Could you check a few things on this model? Use its own coordinates, in mm. Give positions to 0.01 mm unless a question says otherwise; leave off trailing zeros. Loops run counter-clockwise (first coordinate to the right, second up) from the corner with the lowest first, then second, coordinate; pieces in that order, holes last. Notation, with made-up numbers: (-15.5, -14.5) - (22.5, -14.5) arc R24 ccw to (22.5, -4.5) - close; hole circle Ø3 at (55.5, 45.5). An arc over 180 degrees is marked (long way). One line per item, written item: value. Start each with the question number.
Q1. I'm going to push flat-ended pins straight in: P1, Ø4, axis at y = -227.5, z = 155.5, coming from the -X side; P2, Ø2, axis at x = -122.5, z = 405.5, coming from the +Y side; P3, Ø6, axis at x = -8, y = 129.5, coming from the -Z side. Where does each tip first touch, or does it pass through?
Q2. If I drill on line 1 (Z direction, x = 214, y = 232.5); line 2 (X direction, y = -24.5, z = 295.5); line 3 (Y direction, x = -209, z = 122.5), over which ranges is the centre line in solid material (lowest first)? Write a range as from..to.
Q3. I want a section at B-B (x = 51.5). Please give me the cut outline in (y, z).
Q4. If we mould it in two halves opening along Y, with no side actions, what happens to faces 1 (the face through (-10.99, -249.76, 138.75)), 2 (the face through (-74, -239, 12))? For each: released by +Y, released by -Y, zero draft, split by the parting line, or undercut.
Q5. I want a section at C-C (z = 111). Please give me the cut outline in (x, y).
Q6. I want a section at A-A (y = 0). Please give me the cut outline in (x, z).
```python
from build123d import *

# Parameters (mm, degrees)
SKETCH1_R           = 325
SKETCH1_R_2         = 6
SKETCH1_R_3         = 244
BOSS_EXTRUDE1_DEPTH = 12


with BuildPart() as part:
    # Sketch1 → Boss-Extrude1 (new body)
    with BuildSketch(Plane.XY):
        Circle(SKETCH1_R)
        with Locations((0, 287.5)):
            Circle(SKETCH1_R_2, mode=Mode.SUBTRACT)
        with Locations((168.988260034, 232.592385883)):
            Circle(SKETCH1_R_2, mode=Mode.SUBTRACT)
        with Locations((273.428748435, 88.842385883)):
            Circle(SKETCH1_R_2, mode=Mode.SUBTRACT)
        with Locations((273.428748435, -88.842385883)):
            Circle(SKETCH1_R_2, mode=Mode.SUBTRACT)
        with Locations((168.988260034, -232.592385883)):
            Circle(SKETCH1_R_2, mode=Mode.SUBTRACT)
        with Locations((0, -287.5)):
            Circle(SKETCH1_R_2, mode=Mode.SUBTRACT)
        with Locations((-168.988260034, -232.592385883)):
            Circle(SKETCH1_R_2, mode=Mode.SUBTRACT)
        with Locations((-273.428748435, -88.842385883)):
            Circle(SKETCH1_R_2, mode=Mode.SUBTRACT)
        with Locations((-273.428748435, 88.842385883)):
            Circle(SKETCH1_R_2, mode=Mode.SUBTRACT)
        with Locations((-168.988260034, 232.592385883)):
            Circle(SKETCH1_R_2, mode=Mode.SUBTRACT)
        Circle(SKETCH1_R_3, mode=Mode.SUBTRACT)
    extrude(amount=BOSS_EXTRUDE1_DEPTH)

    # Sketch4 → Revolve2 (revolve)
    with BuildSketch(Plane(origin=(0, 0, 0), x_dir=(0, 0, -1), z_dir=(1, 0, 0))):
        with BuildLine():
            Line((-12, 250), (-262, 250))
            ThreePointArc((-262, 250), (-438.776695297, 176.776695297), (-512, 0))
            Line((-512, 0), (-506, 0))
            ThreePointArc((-506, 0), (-434.53405461, 172.53405461), (-262, 244))
            Line((-262, 244), (-12, 244))
            Line((-12, 244), (-12, 250))
        make_face()
    revolve(axis=Axis((0, 0, 12), (0, 0, 1)))


solid = part.part
```
Worked answers:
1. P1: stops at x = -107.93
1. P2: stops at y = 165.16
1. P3: stops at z = 466.73
2. line 1: z = 0..12
2. line 2: x = -246.53..-240.44, 240.44..246.53
2. line 3: y = -137.18..-125.92, 125.92..137.18
3. outline: (-320.89, 0) - (-238.5, 0) - (-238.5, 262) arc R238.5 cw to (238.5, 262) - (238.5, 0) - (320.89, 0) - (320.89, 12) - (244.64, 12) - (244.64, 262) arc R244.64 ccw to (-244.64, 262) - (-244.64, 12) - (-320.89, 12) - close
4. face 1: split by the parting line
4. face 2: zero draft
5. outline: circle Ø500 at (0, 0); hole circle Ø488 at (0, 0)
6. outline: (-325, 0) - (-244, 0) - (-244, 262) arc R244 cw to (244, 262) - (244, 0) - (325, 0) - (325, 12) - (250, 12) - (250, 262) arc R250 ccw to (-250, 262) - (-250, 12) - (-325, 12) - close
